Autodesk Fusion 360 part; units mm, degrees
sketch "スケッチ1" plane through (0, 0, 0) normal (0, 0, 1) x (1, 0, 0)
  line L0 (3, 1.7321) -> (0, 3.4641)
  line L1 (0, 3.4641) -> (-3, 1.7321)
  line L2 (-3, 1.7321) -> (-3, -1.7321)
  line L3 (-3, -1.7321) -> (0, -3.4641)
  line L4 (0, -3.4641) -> (3, -1.7321)
  line L5 (3, -1.7321) -> (3, 1.7321)
  circle A0 centre (0, 0) radius 1.5
extrude "押し出し1" add sketch "スケッチ1" along normal blind 35
sketch "スケッチ2" plane through (0, 0, 35) normal (0, 0, 1) x (-1, 0, 0)
  circle A0 centre (0, 0) radius 1.5
  line L0 (-3, 1.7321) -> (-3, -1.7321)
  line L1 (-3, -1.7321) -> (0, -3.4641)
  line L2 (0, -3.4641) -> (3, -1.7321)
  line L3 (3, -1.7321) -> (3, 1.7321)
  line L4 (3, 1.7321) -> (0, 3.4641)
  line L5 (0, 3.4641) -> (-3, 1.7321)
  line L6 (-3.5, 0) -> (-1.75, -3.0311)
  line L7 (-1.75, -3.0311) -> (1.75, -3.0311)
  line L8 (1.75, -3.0311) -> (3.5, 0)
  line L9 (3.5, 0) -> (1.75, 3.0311)
  line L10 (1.75, 3.0311) -> (-1.75, 3.0311)
  line L11 (-1.75, 3.0311) -> (-3.5, 0)
extrude "押し出し2" add sketch "スケッチ2" along normal blind 4 contours L0 L1 L2 L3 L4 L5 L6 L7 L8 L9 L10 L11 | L0 L6 L11 | L5 L10 L11 | L1 L6 L7 | L4 L9 L10 | L2 L7 L8 | L3 L8 L9
extrude "押し出し3" cut 6 faces at (0, -3.1754, 35) (2.75, -1.5877, 35) (-2.75, -1.5877, 35) (-2.75, 1.5877, 35) (0, 3.1754, 35) (2.75, 1.5877, 35) along direction (0, 0, -1) blind 40
extrude "押し出し4" add 6 faces at (1.5833, 2.7424, 35) (3.1667, 0, 35) (-1.5833, 2.7424, 35) (1.5833, -2.7424, 35) (-1.5833, -2.7424, 35) (-3.1667, 0, 35) along direction (0, 0, -1) blind 35
extrude "押し出し5" cut 1 faces at (2.2005, 1.2273, 39) along direction (0, 0, -1) blind 4
extrude "押し出し6" add 1 faces at (0.0374, 2.5193, 35) along direction (0, 0, 1) blind 10
extrude "押し出し7" add 1 faces at (0.0374, 2.5193, 45) along direction (0, 0, 1) blind 40
extrude "押し出し8" cut 1 faces at (0.0374, 2.5193, 85) along direction (0, 0, -1) blind 50
extrude "押し出し9" add 1 faces at (0.0374, 2.5193, 35) along direction (0, 0, 1) blind 15
Can you work these out from the model? Positions are in its coordinate system, mm. Give positions to 0.01 mm unless a question says otherwise; leave off trailing zeros. Write each loop counter-clockwise with the first axis right and the second up, starting at its lowest first coordinate (ties: lowest second). Pieces come first, ordered by that corner, then holes. Notation, with made-up numbers: (69, 26.5) -> (109, 26.5) arc R5 cw to (109, 30.5) -> close; hole circle Ø1 at (76.5, 76). An arc over 180 degrees is marked (long way). One line per item, written item: value.
Q1. Imagine slicing it at A-A on x = 0. Please give me the cut outline in (y, z).
Results found:
outline: (-3.03, 0) -> (-1.5, 0) -> (-1.5, 50) -> (-3.03, 50) -> close; (1.5, 0) -> (3.03, 0) -> (3.03, 50) -> (1.5, 50) -> close
Q2. Imagine slicing it at C-C on y = 0.5. Please give me the cut outline in (x, z).
Results found:
outline: (-3.21, 0) -> (-1.41, 0) -> (-1.41, 50) -> (-3.21, 50) -> close; (1.41, 0) -> (3.21, 0) -> (3.21, 50) -> (1.41, 50) -> close
Q3. Imagine slicing it at D-D on y = -2.25. Please give me the cut outline in (x, z).
Results found:
outline: (-2.2, 0) -> (2.2, 0) -> (2.2, 50) -> (-2.2, 50) -> close
Q4. Imagine slicing it at B-B on z = 26. Please give me the cut outline in (x, y).
Results found:
outline: (-3.5, 0) -> (-1.75, -3.03) -> (1.75, -3.03) -> (3.5, 0) -> (1.75, 3.03) -> (-1.75, 3.03) -> close; hole circle Ø3 at (0, 0)
Q5. For P1, Ø1.5, axis at y = 1, z = 40.5, coming from the +X side, with a flat end and sliding along its axis, tell me the tip position at first contact or that it passes through.
Results found:
P1: stops at x = 3.36
Q6. We'd pull the mould along X, two halves only. Please class faces 1 (the face through (-2, 0, 50)), 2 (the face through (-1.5, -0.07, 24.65)), 3 (the face through (-2.61, 1.54, 24.65)): +X half, -X half, draft (parallel to the pull), parting line (faces both ways), or undercut.
Results found:
face 1: draft
face 2: undercut
face 3: -X half
Q7. Please list where these lines run through material, in increasing order: line 1 (Y direction, x = 0, z = 17); line 2 (Y direction, x = -0.75, z = 3); line 3 (X direction, y = -1, z = 26). Write a range as [from, to].
Results found:
line 1: y = [-3.03, -1.5], [1.5, 3.03]
line 2: y = [-3.03, -1.3], [1.3, 3.03]
line 3: x = [-2.92, -1.12], [1.12, 2.92]
